For this review, take the finished solid that the model builds, in its own axes (mm). A direction names the side the tool comes from. Give positions to 0.01 mm unless a question says otherwise; leave off trailing zeros. Order: outer loops, then holes, each group sorted by start corner. A loop starts at its lowest first (then second) coordinate and runs counter-clockwise, first axis right, second up.
from build123d import *

# Parameters (mm, degrees)
F1_DEPTH = 63.5
F0_W     = 23.5502142146
F0_H     = 19.05
F0_H_2   = 4.7498
F2_DEPTH = 25.4
F3_DEPTH = 7.9375
F4_R     = 6.35


with BuildPart() as f1:
    # F0 (on Front) → F1 (new body, symmetric)
    with BuildSketch(Plane.XZ):
        Polygon((41.275, -9.525), (41.275, 9.525), (22.225, 9.525), (-41.275, 9.525), (-41.275, -9.525), align=None)
    extrude(amount=F1_DEPTH, both=True)

    # F0 (on Front) → F2 (join, symmetric)
    with BuildSketch(Plane.XZ):
        with BuildLine():
            Line((22.225, 9.525), (41.275, 9.525))
            Line((41.275, 9.525), (41.275, 27.0002))
            ThreePointArc((41.275, 27.0002), (45.9246798487, 38.2255201513), (57.15, 42.8752))
            Line((57.15, 42.8752), (62.6595669536, 42.8752))
            Line((62.6595669536, 42.8752), (62.6595669536, 61.9252))
            Line((62.6595669536, 61.9252), (57.15, 61.9252))
            ThreePointArc((57.15, 61.9252), (32.4542956671, 51.6959043329), (22.225, 27.0002))
            Line((22.225, 27.0002), (22.225, 9.525))
        make_face()
        with Locations((74.4346740609, 52.4002)):
            Rectangle(F0_W, F0_H)
        Polygon((86.2097811682, 61.9252), (86.2097811682, 42.8752), (86.2097811682, 38.1), (108.7904330464, 38.1), (108.7904330464, 66.675), (86.2097811682, 66.675), align=None)
        with Locations((74.4346740609, 64.3001)):
            Rectangle(F0_W, F0_H_2)
    extrude(amount=F2_DEPTH, both=True)

    # F0 (on Front) → F3 (join, symmetric)
    with BuildSketch(Plane.XZ):
        with BuildLine():
            Line((-41.275, 9.525), (22.225, 9.525))
            Line((22.225, 9.525), (22.225, 27.0002))
            ThreePointArc((22.225, 27.0002), (32.4542956671, 51.6959043329), (57.15, 61.9252))
            add(Edge.make_bspline(
                [(-41.275, 9.525), (-37.8933270554, 32.3415985166), (0, 66.4274916053), (57.15, 61.9252)],
                knots=[0, 0, 0, 0, 111.5045361635, 111.5045361635, 111.5045361635, 111.5045361635], degree=3))
        make_face()
    extrude(amount=F3_DEPTH, both=True)

    # F4
    f4_edges = [f1.edges().sort_by_distance(p)[0] for p in [
        (41.275, 63.5, 0),
        (-41.275, 63.5, 0),
        (41.275, -63.5, 0),
        (-41.275, -63.5, 0),
    ]]
    fillet(f4_edges, radius=F4_R)


solid = f1.part
1) We need section A-A on y = -10.5. Give the boundary of the cut face in (x, z) (3 decimals).
Answer sheet:
outline: (-41.275, -9.525) - (41.275, -9.525) - (41.275, 27) arc R15.875 cw to (57.15, 42.875) - (86.21, 42.875) - (86.21, 38.1) - (108.79, 38.1) - (108.79, 66.675) - (62.66, 66.675) - (62.66, 61.925) - (57.15, 61.925) arc R34.925 ccw to (22.225, 27) - (22.225, 9.525) - (-41.275, 9.525) - close
2) Tool access review of faces 1 (the face through (71, 0, 42.875)), 2 (the face through (65, 25.4, 45)), 3 (the face through (97, 0, 38.1)): name each direction out of +Z, -Z, +X, -X, +Y, -Y from which nothing blocks a thin tool from reaching the whole face with its end or side.
Answer sheet:
face 1: -Z, +Y, -Y
face 2: +Z, +X, -X, +Y
face 3: -Z, +X, +Y, -Y
3) To check wall thickness, follow line 1 (Z direction, x = -13.5, y = 56.5) (3 decimals); line 2 (Y direction, x = 43, z = 56); line 3 (X direction, y = -8, z = 41). State the ranges of each line that lie inside material, in increasing order.
Answer sheet:
line 1: z = -9.525 to 9.525
line 2: y = -25.4 to 25.4
line 3: x = 25.15 to 49.67, 86.21 to 108.79
4) Clearance check with flat-ended pins moving along their axes: pin 1 (6 mm diameter, centred on x = 30.5, z = 56.5, fed in from +Y); pin 2 (2 mm diameter, centred on x = 55.5, y = -12.5, fed in from -Z); pin 3 (6 mm diameter, centred on y = -24, z = 44, fed in from -X). State where each tip first meets the part, or that it passes through.
Answer sheet:
pin 1: stops at y = 7.94
pin 2: stops at z = 42.65
pin 3: stops at x = 25.15
5) We need section B-B on x = 64.5. Give the boundary of the cut face in (y, z) (3 decimals).
Answer sheet:
outline: (-25.4, 42.875) - (25.4, 42.875) - (25.4, 66.675) - (-25.4, 66.675) - close
6) Draft analysis for pull direction X (two halves, no side actions). For faces 4 (the face through (39.464, -61.59, 0.133)), 5 (the face through (22.225, -17, 18)), 6 (the face through (45.8, -0.4, 38.1)), state which applies: +X half, -X half, draft (parallel to the pull), parting line (faces both ways), or undercut.
Answer sheet:
face 4: +X half
face 5: -X half
face 6: undercut
7) We need section C-C on y = 49.5. Give the boundary of the cut face in (x, z) (3 decimals).
Answer sheet:
outline: (-41.275, -9.525) - (41.275, -9.525) - (41.275, 9.525) - (-41.275, 9.525) - close
